Input: part model. Units: mm. Frame: model coordinates. A direction names the side the tool comes from. Coordinates: 2 decimals unless noted, no trailing zeros. Order: outer loops, then holes, each group sorted by start corner. A loop starts at its lowest first (then second) coordinate and runs counter-clockwise, first axis right, second up. Notation, with made-up numbers: (56, 47.25) -> (106, 47.25) arc R21 cw to (106, 78.25) -> close; hole circle Ø2 at (38, 66). An arc over 180 degrees is marked (long way). Use one line per item in the form item = value. Start each with the question number.
1) Pin query (flat end, axial travel): pin 1 (0.9 mm diameter, centred on x = -2, z = 2, fed in from +Y); pin 2 (0.9 mm diameter, centred on y = -0.5, z = 1.5, fed in from +X); pin 3 (0.9 mm diameter, centred on y = -3, z = 2, fed in from -X). Return the tip coordinate at first contact, or that it passes through.
2) Section query C-C on y = -16. Output: boundary loops of the cut face in (x, z).
3) Draft query along X for faces 6 (the flat face through (-2, -4, 1)), 7 (the flat face through (124, -2, 1)), 8 (the flat face through (86.05, -3, 2)). Return one class per face: pulls with the +X half, pulls with the -X half, needs draft (parallel to the pull), parting line crosses it, or undercut.
4) Section query B-B on x = 18. Output: boundary loops of the cut face in (y, z).
5) Ray query, line 1 along X through (y, z) = (-6, 0.3); line 2 along X through (y, z) = (-0.5, 2.65); line 3 along Y through (x, z) = (97, 0.25). Return the intervals inside material, ascending.
6) Section query A-A on z = 1.55. Output: boundary loops of the cut face in (x, y), then the cut area to 3 significant figures.
7) Access query for faces 1 (the flat face through (0, -15, 1)), 2 (the flat face through (126, -4, 1)), 3 (the flat face through (17, 0, 1)), 4 (the flat face through (125, -12, 1)), 5 (the flat face through (35, -4, 1)). Directions: +Z, -Z, +X, -X, +Y, -Y. A direction counts if a zero-diameter tool reaches every point of the face in a straight line with its end or side. Return the directions, or none.
Autodesk Inventor part; units mm, degrees
ref_plane "YZ Plane" through (0, 0, 0) normal (1, 0, 0) x (0, 1, 0)
ref_plane "XZ Plane" through (0, 0, 0) normal (0, 1, 0) x (-1, 0, 0)
ref_plane "XY Plane" through (0, 0, 0) normal (0, 0, 1) x (1, 0, 0)
sketch "草圖1" plane through (0, 0, 0) normal (0, 0, 1) x (1, 0, 0)
  line L0 (0, 0) -> (124, 0)
  line L1 (124, 0) -> (124, -18) construction
  line L2 (124, -18) -> (0, -18)
  line L3 (0, -18) -> (0, 0) construction
  line L4 (35, 0) -> (37.95, 0)
  line L5 (37.95, 0) -> (37.95, -7.5)
  line L6 (37.95, -7.5) -> (35, -7.5)
  line L7 (35, -7.5) -> (35, 0)
  line L8 (89, 0) -> (86.05, 0)
  line L9 (86.05, 0) -> (86.05, -7.5)
  line L10 (86.05, -7.5) -> (89, -7.5)
  line L11 (89, -7.5) -> (89, 0)
  line L12 (0, -18) -> (0, 0) construction
  line L13 (-3, -12) -> (0, -12)
  line L14 (0, -12) -> (0, -18)
  line L15 (124, -12) -> (124, -18)
  line L16 (-3, -12) -> (-3, -4)
  line L17 (-3, -4) -> (0, -4)
  line L18 (0, 0) -> (0, -4)
  line L19 (124, -12) -> (127, -12)
  line L20 (127, -12) -> (127, -4)
  line L21 (127, -4) -> (124, -4)
  line L22 (124, -4) -> (124, -12)
  line L23 (124, 0) -> (124, -4)
  point P0 (0, -15.5)
  dimension "d0" = 124
  dimension "d1" = 35
  dimension "d3" = 2.95
  dimension "d4" = 2.95
  dimension "d10" = 10.5
  dimension "d16" = 7.5
  dimension "d17" = 35
  dimension "d29" = 8
  dimension "d30" = 4
  dimension "d31" = 3
  dimension "d32" = 3
  dimension "d33" = 4
  dimension "d34" = 8
extrude "擠出1" add sketch "草圖1" along normal blind 3 contours L0 L7 L6 L5 L9 L10 L11 L23 L22 L15 L2 L14 L13 L16 L17 L18 | L21 L20 L19 L22
sketch "草圖2" plane through (0, 0, 3) normal (0, 0, 1) x (1, 0, 0)
  line L0 (37.95, 0) -> (86.05, 0)
  line L1 (86.05, 0) -> (86.05, 2)
  line L2 (86.05, 2) -> (37.95, 2)
  line L3 (37.95, 2) -> (37.95, 0)
  line L4 (86.05, -7.5) -> (86.05, 0)
  point P0 (0, 0)
  dimension "d26" = 2
extrude "擠出2" add sketch "草圖2" against normal up to surface (3 mm away)
sketch "草圖3" plane through (0, 0, 3) normal (0, 0, 1) x (1, 0, 0)
  line L0 (124, 0) -> (89, 0)
  line L1 (89, 0) -> (89, -7.5)
  line L2 (89, -7.5) -> (86.05, -7.5)
  line L3 (86.05, -7.5) -> (86.05, 2)
  line L4 (37.95, -7.5) -> (35, -7.5)
  line L5 (35, -7.5) -> (35, 0)
  line L6 (35, 0) -> (0, 0)
  line L7 (0, -4) -> (-3, -4)
  line L8 (-3, -4) -> (-3, -12)
  line L9 (-3, -12) -> (0, -12)
  line L10 (0, -12) -> (0, -18)
  line L11 (0, -18) -> (124, -18)
  line L12 (124, -18) -> (124, -12)
  line L13 (124, -12) -> (127, -12)
  line L14 (127, -12) -> (127, -4)
  line L15 (127, -4) -> (124, -4)
  line L16 (124, -4) -> (124, 0)
  line L17 (86.05, 2) -> (37.95, 2)
  line L18 (37.95, 2) -> (37.95, -7.5)
  line L19 (0, 0) -> (0, -4)
properties part number "chassis_1_6"
Answers below:
q1.pin_1 = -4
q1.pin_2 = 124
q1.pin_3 = 0
q2.outline = (0, 0) -> (124, 0) -> (124, 3) -> (0, 3) -> close
q3.face_6 = needs draft
q3.face_7 = pulls with the +X half
q3.face_8 = undercut
q4.outline = (-18, 0) -> (0, 0) -> (0, 3) -> (-18, 3) -> close
q5.line_1 = -3 to 35, 37.95 to 86.05, 89 to 127
q5.line_2 = 0 to 35, 37.95 to 86.05, 89 to 124
q5.line_3 = -18 to 0
q6.outline = (-3, -12) -> (0, -12) -> (0, -18) -> (124, -18) -> (124, -12) -> (127, -12) -> (127, -4) -> (124, -4) -> (124, 0) -> (89, 0) -> (89, -7.5) -> (86.05, -7.5) -> (86.05, 2) -> (37.95, 2) -> (37.95, -7.5) -> (35, -7.5) -> (35, 0) -> (0, 0) -> (0, -4) -> (-3, -4) -> close
q6.area = 2,330 mm^2
q7.face_1 = +Z, -Z, -X, -Y
q7.face_2 = +Z, -Z, +X, +Y
q7.face_3 = +Z, -Z, -X, +Y
q7.face_4 = +Z, -Z, +X, -Y
q7.face_5 = +Z, -Z, +Y
